```python
from build123d import *

# Parameters (mm, degrees)
SKETCH1_R           = 30.675
SKETCH1_R_2         = 2
SKETCH1_R_3         = 20
BOSS_EXTRUDE1_DEPTH = 5
CHAMFER6_SIZE       = 1
CHAMFER6_SIZE2      = 2.144506921


with BuildPart() as part:
    # Sketch1 → Boss-Extrude1 (new body)
    with BuildSketch(Plane.XY):
        Circle(SKETCH1_R)
        with Locations((0, 24)):
            Circle(SKETCH1_R_2, mode=Mode.SUBTRACT)
        Circle(SKETCH1_R_3, mode=Mode.SUBTRACT)
        with Locations((20.784609691, 12)):
            Circle(SKETCH1_R_2, mode=Mode.SUBTRACT)
        with Locations((20.784609691, -12)):
            Circle(SKETCH1_R_2, mode=Mode.SUBTRACT)
        with Locations((0, -24)):
            Circle(SKETCH1_R_2, mode=Mode.SUBTRACT)
        with Locations((-20.784609691, -12)):
            Circle(SKETCH1_R_2, mode=Mode.SUBTRACT)
        with Locations((-20.784609691, 12)):
            Circle(SKETCH1_R_2, mode=Mode.SUBTRACT)
    extrude(amount=BOSS_EXTRUDE1_DEPTH)

    # Chamfer6
    chamfer6_edges = [part.edges().sort_by_distance(p)[0] for p in [
        (-30.675, 0, 0),
        (-20, 0, 0),
    ]]
    chamfer6_side = [part.faces().sort_by_distance(p)[0] for p in [
        (-29.807379979, 0, 0),
    ]]
    chamfer(chamfer6_edges, length=CHAMFER6_SIZE, length2=CHAMFER6_SIZE2, reference=chamfer6_side[0])


solid = part.part
```
The model under review builds one solid part; all positions refer to its coordinate system, in mm. Coordinates: 2 decimals unless noted, no trailing zeros. Loops run counter-clockwise (first coordinate to the right, second up) from the corner with the lowest first, then second, coordinate; pieces in that order, holes last. Notation, with made-up numbers: (-2, 81.5) -> (13, 81.5) arc R34 cw to (13, 118.5) -> close; hole circle Ø2 at (65, 25). An arc over 180 degrees is marked (long way). Answer as CSV lines item,"result".
Item 1: Take a section at A-A, the plane x = 0. State the section outline as (y, z) points (1 decimal), and give its area (3 significant figures).
Results below:
outline,"(-30.7, 2.1) -> (-29.7, 0) -> (-26, 0) -> (-26, 5) -> (-30.7, 5) -> close; (-22, 0) -> (-21, 0) -> (-20, 2.1) -> (-20, 5) -> (-22, 5) -> close; (20, 2.1) -> (21, 0) -> (22, 0) -> (22, 5) -> (20, 5) -> close; (26, 0) -> (29.7, 0) -> (30.7, 2.1) -> (30.7, 5) -> (26, 5) -> close"
area,"62.5 mm2"
Item 2: Take a section at C-C, the plane y = 0. State the section outline as (x, z) points (1 decimal).
Results below:
outline,"(-30.7, 2.1) -> (-29.7, 0) -> (-21, 0) -> (-20, 2.1) -> (-20, 5) -> (-30.7, 5) -> close; (20, 2.1) -> (21, 0) -> (29.7, 0) -> (30.7, 2.1) -> (30.7, 5) -> (20, 5) -> close"
Item 3: Insertion check: pin 1 (8 mm diameter, centred on x = 14.5, y = -13, fed in from +Z); pin 2 (1 mm diameter, centred on x = -1.5, z = 2.5, fed in from +Y); pin 3 (3 mm diameter, centred on x = -20.5, z = 3.5, fed in from +Y). Each pin has a flat end and moves straight along its axis. Give the tip position at first contact, or say it passes through.
Results below:
pin 1,"stops at z = 5"
pin 2,"stops at y = 30.66"
pin 3,"stops at y = 24.08"
Item 4: Take a section at D-D, the plane x = -22. Count the separate pieces of the cut face and the enclosed holes in it, and give its area (3 significant figures).
Results below:
separate pieces,"3"
enclosed holes,"0"
area,"179 mm2"
Item 5: Take a section at B-B, the plane z = 3.15. State the section outline as (x, y) points (3 decimals), and give its area (3 significant figures).
Results below:
outline,"circle Ø61.35 at (0, 0); hole circle Ø4 at (-20.785, -12); hole circle Ø4 at (-20.785, 12); hole circle Ø40 at (0, 0); hole circle Ø4 at (0, -24); hole circle Ø4 at (0, 24); hole circle Ø4 at (20.785, -12); hole circle Ø4 at (20.785, 12)"
area,"1,620 mm2"
Item 6: For L1, parallel to Y at x = 0, z = 2.3 (3 decimals); L2, parallel to X at y = 0.5, z = 3.45; L3, parallel to Y at x = -21, z = 0.8, list the stretches that pass through material, from the lowest coordinate up.
Results below:
L1,"y = -30.675 to -26, -22 to -20, 20 to 22, 26 to 30.675"
L2,"x = -30.67 to -19.99, 19.99 to 30.67"
L3,"y = -21.49 to -13.99, -10.01 to 10.01, 13.99 to 21.49"
Item 7: Draft analysis for pull direction X (two halves, no side actions). For faces 1 (the cylindrical face through (20.524, 13.983, 2.465)), 2 (the cylindrical face through (-30.645, 1.349, 3.552)), 3 (the flat face through (20, -6, 5)), 4 (the cylindrical face through (0.923, 22.226, 2.465)), state which applies: +X half, -X half, draft (parallel to the pull), parting line (faces both ways), or undercut.
Results below:
face 1,"undercut"
face 2,"parting line"
face 3,"draft"
face 4,"undercut"
